CAD build for the part. Positions are in the model's coordinates, mm. Coordinates: 2 decimals unless noted, no trailing zeros. Order: outer loops, then holes, each group sorted by start corner. A loop starts at its lowest first (then second) coordinate and runs counter-clockwise, first axis right, second up. Notation, with made-up numbers: (7.5, 23) - (56.5, 23) arc R22 ccw to (56.5, 30) - close; hole circle Ø5 at (80.25, -31.75). An arc over 180 degrees is marked (long way). Return JSON: item names as keys, results as strings.
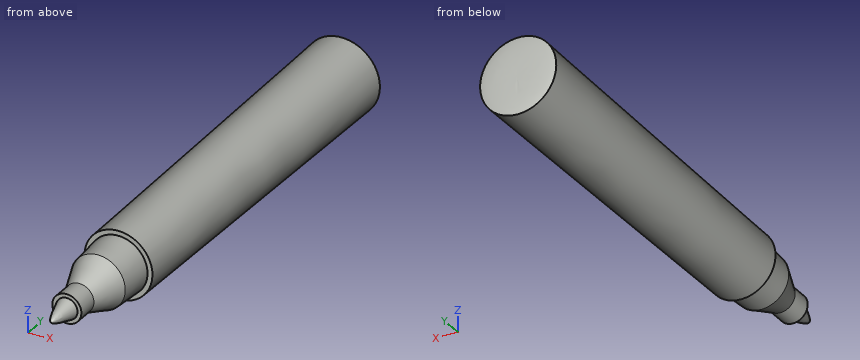
from build123d import *


with BuildPart() as part:
    # Sketch1 → Revolve1 (revolve)
    with BuildSketch(Plane.XY, mode=Mode.PRIVATE) as revolve1_sk:
        with BuildLine():
            Line((0, 0), (0, 130))
            add(Edge.make_bspline(
                [(0, 130), (7.444716878, 130.087394751), (9.95, 129.5)],
                knots=[0, 0, 0, 1, 1, 1], degree=2))
            Line((9.95, 129.5), (8.875, 30))
            Line((8.875, 30), (7.6, 30))
            Line((7.6, 30), (7.05, 21))
            Line((7.05, 21), (3.8, 12.6))
            Line((3.8, 12.6), (3.8, 7))
            Line((3.8, 7), (2.8, 7))
            add(Edge.make_bspline(
                [(0, 0), (0.934954865, 0.032949741), (2.8, 7)],
                knots=[0, 0, 0, 1, 1, 1], degree=2))
        make_face()
    revolve(revolve1_sk.sketch.rotate(Axis((0, 0, 0), (0, 1, 0)), 90), axis=Axis((0, 0, 0), (0, 1, 0)))


solid = part.part
Item 1: Wall check: L1, parallel to X at y = 115, z = -3.5; L2, parallel to Z at x = 7.75, y = 36; L3, parallel to Y at x = 4.25, z = -2.25. Give the ranges that are in metal, low to high. Write a range as [from, to].
Findings below:
{"L1": "x = [-9.15, 9.15]", "L2": "z = [-4.46, 4.46]", "L3": "y = [15.21, 129.97]"}
Item 2: Band-saw the part on B-B, the plane y = 58. List the corners of the cut face in (x, z), then the cut area to 3 significant figures.
Findings below:
{"outline": "circle Ø18.36 at (0, 0)", "area": "265 mm²"}
Item 3: Band-saw the part on A-A, the plane y = 111. List the corners of the cut face in (x, z), then the cut area to 3 significant figures.
Findings below:
{"outline": "circle Ø19.5 at (0, 0)", "area": "299 mm²"}
Item 4: Drop flat-ended pins along their axis: P1, Ø8, axis at x = 8, y = 98.5, coming from the -Z side; P2, Ø6, axis at y = 95.5, z = -1.5, coming from the +X side; P3, Ø10, axis at y = 101.5, z = 1.5, coming from the +X side. Give the stop position or say it passes through.
Findings below:
{"P1": "stops at z = -8.74", "P2": "stops at x = 9.61", "P3": "stops at x = 9.7"}
